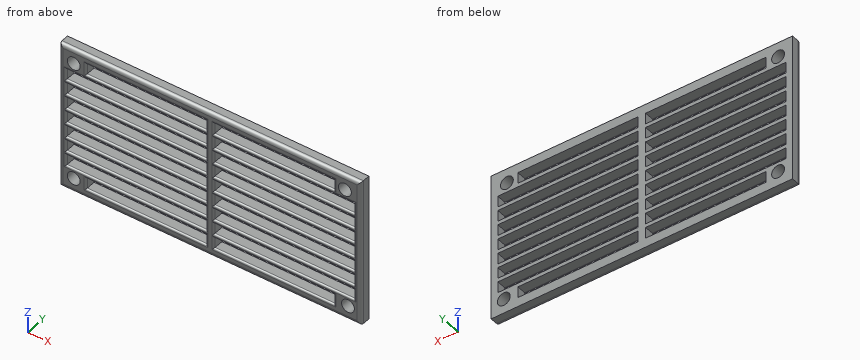
```python
from build123d import *

# Parameters (mm, degrees)
F0_W     = 82
F0_H     = 40
F0_R     = 1.75
F0_W_2   = 2.0507176579
F0_H_2   = 3
F0_H_3   = 1
F1_DEPTH = 3
F2_R     = 0.49999
F3_R     = 1


# Not quite as in the source:
# - a fillet or chamfer is up to 0.001 mm smaller than in the source, because OpenCascade refuses the exact size


with BuildPart() as f1:
    # F0 (on Front) → F1 (new body)
    with BuildSketch(Plane.XZ):
        with Locations((-54.7693173022, 38.4868923018)):
            Rectangle(F0_W, F0_H)
        with Locations((-91.8560757875, 22.4002130298)):
            Circle(F0_R, mode=Mode.SUBTRACT)
        with Locations((-17.2127172435, 22.4002130298)):
            Circle(F0_R, mode=Mode.SUBTRACT)
        with Locations((-91.8560757875, 54.5735715738)):
            Circle(F0_R, mode=Mode.SUBTRACT)
        Polygon((-53.7439584732, 39.9868923018), (-15.5743994219, 39.9868923018), (-15.5743994219, 36.9868923018), (-53.7439584732, 36.9868923018), (-53.7439584732, 35.9868923018), (-15.5743994219, 35.9868923018), (-15.5743994219, 32.9868923018), (-53.7439584732, 32.9868923018), (-53.7439584732, 31.9868923018), (-15.5743994219, 31.9868923018), (-15.5743994219, 28.9868923018), (-53.7439584732, 28.9868923018), (-53.7439584732, 27.9868923018), (-15.5743994219, 27.9868923018), (-15.5743994219, 24.9868923018), (-53.7439584732, 24.9868923018), (-53.7439584732, 23.9868923018), (-21.0193173022, 23.9868923018), (-21.0193173022, 20.9868923018), (-53.7439584732, 20.9868923018), (-55.7946761312, 20.9868923018), (-88.5193173022, 20.9868923018), (-88.5193173022, 23.9868923018), (-55.7946761312, 23.9868923018), (-55.7946761312, 24.9868923018), (-93.9642351825, 24.9868923018), (-93.9642351825, 27.9868923018), (-55.7946761312, 27.9868923018), (-55.7946761312, 28.9868923018), (-93.9642351825, 28.9868923018), (-93.9642351825, 31.9868923018), (-55.7946761312, 31.9868923018), (-55.7946761312, 32.9868923018), (-93.9642351825, 32.9868923018), (-93.9642351825, 35.9868923018), (-55.7946761312, 35.9868923018), (-55.7946761312, 36.9868923018), (-93.9642351825, 36.9868923018), (-93.9642351825, 39.9868923018), (-55.7946761312, 39.9868923018), (-55.7946761312, 40.9868923018), (-93.9642351825, 40.9868923018), (-93.9642351825, 43.9868923018), (-55.7946761312, 43.9868923018), (-55.7946761312, 44.9868923018), (-93.9642351825, 44.9868923018), (-93.9642351825, 47.9868923018), (-55.7946761312, 47.9868923018), (-55.7946761312, 48.9868923018), (-93.9642351825, 48.9868923018), (-93.9642351825, 51.9868923018), (-55.7946761312, 51.9868923018), (-55.7946761312, 52.9868923018), (-88.5193173022, 52.9868923018), (-88.5193173022, 55.9868923018), (-55.7946761312, 55.9868923018), (-53.7439584732, 55.9868923018), (-21.0193173022, 55.9868923018), (-21.0193173022, 52.9868923018), (-53.7439584732, 52.9868923018), (-53.7439584732, 51.9868923018), (-15.5743994219, 51.9868923018), (-15.5743994219, 48.9868923018), (-53.7439584732, 48.9868923018), (-53.7439584732, 47.9868923018), (-15.5743994219, 47.9868923018), (-15.5743994219, 44.9868923018), (-53.7439584732, 44.9868923018), (-53.7439584732, 43.9868923018), (-15.5743994219, 43.9868923018), (-15.5743994219, 40.9868923018), (-53.7439584732, 40.9868923018), align=None, mode=Mode.SUBTRACT)
        with Locations((-18.0520743152, 54.5735715738)):
            Circle(F0_R, mode=Mode.SUBTRACT)
        with Locations((-54.7693173022, 54.4868923018)):
            Rectangle(F0_W_2, F0_H_2)
        with Locations((-54.7693173022, 52.4868923018)):
            Rectangle(F0_W_2, F0_H_3)
        with Locations((-54.7693173022, 50.4868923018)):
            Rectangle(F0_W_2, F0_H_2)
        with Locations((-54.7693173022, 48.4868923018)):
            Rectangle(F0_W_2, F0_H_3)
        with Locations((-54.7693173022, 46.4868923018)):
            Rectangle(F0_W_2, F0_H_2)
        with Locations((-54.7693173022, 44.4868923018)):
            Rectangle(F0_W_2, F0_H_3)
        with Locations((-54.7693173022, 42.4868923018)):
            Rectangle(F0_W_2, F0_H_2)
        with Locations((-54.7693173022, 40.4868923018)):
            Rectangle(F0_W_2, F0_H_3)
        with Locations((-54.7693173022, 38.4868923018)):
            Rectangle(F0_W_2, F0_H_2)
        with Locations((-54.7693173022, 36.4868923018)):
            Rectangle(F0_W_2, F0_H_3)
        with Locations((-54.7693173022, 34.4868923018)):
            Rectangle(F0_W_2, F0_H_2)
        with Locations((-54.7693173022, 32.4868923018)):
            Rectangle(F0_W_2, F0_H_3)
        with Locations((-54.7693173022, 30.4868923018)):
            Rectangle(F0_W_2, F0_H_2)
        with Locations((-54.7693173022, 28.4868923018)):
            Rectangle(F0_W_2, F0_H_3)
        with Locations((-54.7693173022, 26.4868923018)):
            Rectangle(F0_W_2, F0_H_2)
        with Locations((-54.7693173022, 24.4868923018)):
            Rectangle(F0_W_2, F0_H_3)
        with Locations((-54.7693173022, 22.4868923018)):
            Rectangle(F0_W_2, F0_H_2)
    extrude(amount=F1_DEPTH)

    # F2 (radius 0.5 in the source; OpenCascade refuses exactly that, so slightly less here)
    f2_edges = [f1.edges().sort_by_distance(p)[0] for p in [
        (-72.156997, -3, 20.986892),
        (-72.156997, -3, 23.986892),
        (-74.879456, -3, 24.986892),
        (-74.879456, -3, 27.986892),
        (-74.879456, -3, 28.986892),
        (-74.879456, -3, 31.986892),
        (-74.879456, -3, 32.986892),
        (-74.879456, -3, 35.986892),
        (-74.879456, -3, 36.986892),
        (-37.381638, -3, 20.986892),
        (-37.381638, -3, 23.986892),
        (-34.659179, -3, 24.986892),
        (-34.659179, -3, 27.986892),
        (-34.659179, -3, 28.986892),
        (-34.659179, -3, 31.986892),
        (-34.659179, -3, 32.986892),
        (-34.659179, -3, 35.986892),
        (-34.659179, -3, 36.986892),
        (-74.879456, -3, 39.986892),
        (-74.879456, -3, 40.986892),
        (-74.879456, -3, 43.986892),
        (-74.879456, -3, 44.986892),
        (-74.879456, -3, 47.986892),
        (-74.879456, -3, 48.986892),
        (-74.879456, -3, 51.986892),
        (-72.156997, -3, 52.986892),
        (-93.964235, -3, 26.486892),
        (-93.964235, -3, 30.486892),
        (-93.964235, -3, 34.486892),
        (-88.519317, -3, 22.486892),
        (-55.794676, -3, 22.486892),
        (-55.794676, -3, 26.486892),
        (-55.794676, -3, 30.486892),
        (-55.794676, -3, 34.486892),
        (-55.794676, -3, 38.486892),
        (-55.794676, -3, 42.486892),
        (-55.794676, -3, 46.486892),
        (-55.794676, -3, 50.486892),
        (-55.794676, -3, 54.486892),
        (-72.156997, -3, 55.986892),
        (-53.743958, -3, 22.486892),
        (-53.743958, -3, 26.486892),
        (-53.743958, -3, 30.486892),
        (-53.743958, -3, 34.486892),
        (-53.743958, -3, 38.486892),
        (-34.659179, -3, 39.986892),
        (-34.659179, -3, 40.986892),
        (-53.743958, -3, 42.486892),
        (-34.659179, -3, 43.986892),
        (-34.659179, -3, 44.986892),
        (-53.743958, -3, 46.486892),
        (-34.659179, -3, 48.986892),
        (-34.659179, -3, 47.986892),
        (-53.743958, -3, 50.486892),
        (-34.659179, -3, 51.986892),
        (-37.381638, -3, 52.986892),
        (-53.743958, -3, 54.486892),
        (-37.381638, -3, 55.986892),
        (-93.964235, -3, 38.486892),
        (-93.964235, -3, 42.486892),
        (-93.964235, -3, 46.486892),
        (-93.964235, -3, 50.486892),
        (-88.519317, -3, 54.486892),
        (-21.019317, -3, 22.486892),
        (-15.574399, -3, 26.486892),
        (-15.574399, -3, 30.486892),
        (-15.574399, -3, 34.486892),
        (-15.574399, -3, 38.486892),
        (-15.574399, -3, 42.486892),
        (-15.574399, -3, 46.486892),
        (-15.574399, -3, 50.486892),
        (-21.019317, -3, 54.486892),
    ]]
    fillet(f2_edges, radius=F2_R)

    # F3
    f3_edges = [f1.edges().sort_by_distance(p)[0] for p in [
        (-54.769317, -3, 58.486892),
        (-13.769317, -3, 38.486892),
        (-54.769317, -3, 18.486892),
        (-95.769317, -3, 38.486892),
    ]]
    fillet(f3_edges, radius=F3_R)


solid = f1.part
```
Model file for the job. Use its own axes, mm. Coordinates: 2 decimals unless noted, no trailing zeros. Order: outer loops, then holes, each group sorted by start corner. A loop starts at its lowest first (then second) coordinate and runs counter-clockwise, first axis right, second up. Notation, with made-up numbers: (13.25, -10.75) - (51.25, -10.75) arc R21 cw to (51.25, 15.25) - close; hole circle Ø10 at (54, 41). An arc over 180 degrees is marked (long way). Return JSON: item names as keys, results as strings. Group by question number.
1) Flat gauge pin, fed straight in: P1, Ø3, axis at x = -91.86, z = 54.57, coming from the -Y side. Where does the tip first touch, or does it go through?
2) Saw through at B-B, the plane x = -24. Count the separate pieces of the cut face and the enclosed holes in it, plus the area to 3 significant figures.
3) Probe line 1 (X direction, y = -0.75, z = 35.5); line 2 (X direction, y = -2.55, z = 34); line 3 (X direction, y = -0.6, z = 55.5). List the from-to ranges inside material, lowest first. Write a range as from..to.
4) Saw through at A-A, the plane z = 42. Write the cut outline in (x, y), plus the area to 3 significant figures.
Values found:
{
 "1": {"P1": "passes through"},
 "2": {"separate pieces": "10", "enclosed holes": "0", "area": "37.6 mm²"},
 "3": {"line 1": "x = -95.77..-93.96, -55.79..-53.74, -15.57..-13.77", "line 2": "x = -95.6..-93.97, -55.79..-53.75, -15.57..-13.93", "line 3": "x = -95.77..-93.34, -90.37..-88.52, -55.79..-53.74, -21.02..-19.54, -16.57..-13.77"},
 "4": {"outline": "(-95.77, -2) arc R1 ccw to (-94.77, -3) - (-94.46, -3) arc R0.5 ccw to (-93.96, -2.5) - (-93.96, 0) - (-95.77, 0) - close; (-55.79, -2.5) arc R0.5 ccw to (-55.29, -3) - (-54.24, -3) arc R0.5 ccw to (-53.74, -2.5) - (-53.74, 0) - (-55.79, 0) - close; (-15.57, -2.5) arc R0.5 ccw to (-15.07, -3) - (-14.77, -3) arc R1 ccw to (-13.77, -2) - (-13.77, 0) - (-15.57, 0) - close", "area": "16.3 mm²"}
}
